```python
from build123d import *

# Parameters (mm, degrees)
F0_W            = 305
F0_H            = 200
F1_DEPTH        = 25
F3_D            = 11
F3_CSINK_D      = 11.25
F3_CSINK_ANGLE  = 90
F5_DEPTH        = 152.501
F5_DEPTH_BACK   = 152.501
F6_SIZE         = 1
F10_D           = 6.35
F10_DEPTH       = 42
F10_TIP         = 1.9077324654
F11_D           = 6.35
F11_DEPTH       = 57
F11_TIP         = 1.9077324654
F11_ON_F8_D     = 6.35
F11_ON_F8_DEPTH = 57
F11_ON_F8_TIP   = 1.9077324654


with BuildPart() as f1:
    # F0 (on Top) → F1 (new body)
    with BuildSketch(Plane.XY):
        Rectangle(F0_W, F0_H)
    extrude(amount=-F1_DEPTH)

    # F3 (through all)
    with Locations(Plane.XY):
        with Locations((-137.5, 75), (137.5, 75), (137.5, -75), (-137.5, -75)):
            CounterSinkHole(F3_D / 2, F3_CSINK_D / 2, counter_sink_angle=F3_CSINK_ANGLE)

    # F4 (on Right) → F5 (cut, two sides)
    with BuildSketch(Plane.YZ) as f5_sk:
        Polygon((-34.75, 0), (-40, 0), (-45.25, 0), (-45.25, -6.5), (-48.25, -6.5), (-48.25, -13.5), (-40, -13.5), (-31.75, -13.5), (-31.75, -6.5), (-34.75, -6.5), align=None)
        Polygon((65.25, 0), (60, 0), (54.75, 0), (54.75, -6.5), (51.75, -6.5), (51.75, -13.5), (60, -13.5), (68.25, -13.5), (68.25, -6.5), (65.25, -6.5), align=None)
    extrude(amount=-F5_DEPTH, mode=Mode.SUBTRACT)
    extrude(f5_sk.sketch, amount=F5_DEPTH_BACK, mode=Mode.SUBTRACT)

    # F6
    f6_edges = [f1.edges().sort_by_distance(p)[0] for p in [
        (0, -34.75, 0),
        (0, -45.25, 0),
        (0, 65.25, 0),
        (0, 54.75, 0),
    ]]
    chamfer(f6_edges, length=F6_SIZE)

    # F10
    with Locations(Plane.XZ.offset(100)):
        with Locations((97.5, -12.5), (-97.5, -12.5)):
            Hole(F10_D / 2, depth=F10_DEPTH)
            with Locations((0, 0, -(F10_DEPTH + F10_TIP / 2))):  # 118° drill point
                Cone(0, F10_D / 2, F10_TIP, mode=Mode.SUBTRACT)

    # F11
    with Locations(Plane(origin=(-152.5, 0, 0), x_dir=(0, -1, 0), z_dir=(-1, 0, 0))):
        with Locations((60, -12.5)):
            Hole(F11_D / 2, depth=F11_DEPTH)
            with Locations((0, 0, -(F11_DEPTH + F11_TIP / 2))):  # 118° drill point
                Cone(0, F11_D / 2, F11_TIP, mode=Mode.SUBTRACT)

    # F11 on F8
    with Locations(Plane.YZ.offset(152.5)):
        with Locations((-60, -12.5)):
            Hole(F11_ON_F8_D / 2, depth=F11_ON_F8_DEPTH)
            with Locations((0, 0, -(F11_ON_F8_DEPTH + F11_ON_F8_TIP / 2))):  # 118° drill point
                Cone(0, F11_ON_F8_D / 2, F11_ON_F8_TIP, mode=Mode.SUBTRACT)


solid = f1.part
```
Work out the finished part from the listing and answer in its coordinate system (mm). A direction names the side the tool comes from. Coordinates: 2 decimals unless noted, no trailing zeros. Loops run counter-clockwise (first coordinate to the right, second up) from the corner with the lowest first, then second, coordinate; pieces in that order, holes last.
1) Flat-ended cylindrical pins translate along their axes: pin 1 (5 mm diameter, centred on y = -60, z = -12.5, fed in from -X); pin 2 (2 mm diameter, centred on x = 95.5, z = -12.5, fed in from -Y); pin 3 (5 mm diameter, centred on x = 14, y = -38.5, fed in from +Z); pin 4 (9 mm diameter, centred on x = 137.5, y = -75, fed in from +Z). Find the tip coordinate at first contact, or state that the pin passes through.
Results:
pin 1: stops at x = -95.09
pin 2: stops at y = -57.89
pin 3: stops at z = -13.5
pin 4: passes through
2) For faces 5 (the cylindrical face through (124.62, -56.83, -12.36)), 6 (the flat face through (2, -34.75, -4)), 7 (the cylindrical face through (-124.62, -57.07, -13.72)), 8 (the flat face through (2, -40, -13.5)), 9 (the cylindrical face through (-94.33, -79.72, -12.36)), determine the directions among +Z, -Z, +X, -X, +Y, -Y from which every point of the face is accessible in a straight line to the end or side of a thin tool.
Results:
face 5: +X
face 6: +Z, +X, -X
face 7: -X
face 8: +X, -X
face 9: -Y
3) Section D-D (y = 60) is taken. Give the vertices of the cut face in (x, z), plus the area to 3 significant figures.
Results:
outline: (-152.5, -25) - (152.5, -25) - (152.5, -13.5) - (-152.5, -13.5) - close
area: 3,510 mm2
4) Section C-C (x = 14.5) is taken. Give the vertices of the cut face in (y, z).
Results:
outline: (-100, -25) - (100, -25) - (100, 0) - (66.25, 0) - (65.25, -1) - (65.25, -6.5) - (68.25, -6.5) - (68.25, -13.5) - (51.75, -13.5) - (51.75, -6.5) - (54.75, -6.5) - (54.75, -1) - (53.75, 0) - (-33.75, 0) - (-34.75, -1) - (-34.75, -6.5) - (-31.75, -6.5) - (-31.75, -13.5) - (-48.25, -13.5) - (-48.25, -6.5) - (-45.25, -6.5) - (-45.25, -1) - (-46.25, 0) - (-100, 0) - close
5) Consider probe 1 along X at (y, z) = (75, -13.5); probe 2 along Y at (x, z) = (-36.5, -7); probe 3 along Y at (x, z) = (-22, -5.25). Determine where each line is inside the solid, lowest interval first.
Results:
probe 1: x = -152.5 to -143, -132 to 132, 143 to 152.5
probe 2: y = -100 to -48.25, -31.75 to 51.75, 68.25 to 100
probe 3: y = -100 to -45.25, -34.75 to 54.75, 65.25 to 100
6) Section B-B (x = 137.5) is taken. Give the number of separate pieces and of enclosed holes in the cut face, plus the area to 3 significant figures.
Results:
separate pieces: 3
enclosed holes: 1
area: 4,050 mm2
7) For a pull along X with two mould halves and no side action, classify faces 1 (the flat face through (152.5, -1, -12)), 2 (the cylindrical face through (-132, -75, -13)), 3 (the cylindrical face through (94.47, -79.72, -11.55)), 4 (the flat face through (-2, 11, 0)) as +X half, -X half, draft (parallel to the pull), parting line (faces both ways), or undercut.
Results:
face 1: +X half
face 2: undercut
face 3: undercut
face 4: draft
8) Section A-A (y = -75) is taken. Give the vertices of the cut face in (x, z) (3 decimals), plus the area to 3 significant figures.
Results:
outline: (-152.5, -25) - (-143, -25) - (-143, -0.125) - (-143.125, 0) - (-152.5, 0) - close; (-132, -25) - (132, -25) - (132, -0.125) - (131.875, 0) - (-131.875, 0) - (-132, -0.125) - close; (143, -25) - (152.5, -25) - (152.5, 0) - (143.125, 0) - (143, -0.125) - close; hole circle Ø6.35 at (-97.5, -12.5); hole circle Ø6.35 at (97.5, -12.5)
area: 7,010 mm2
